```python
from build123d import *

# Parameters (mm, degrees)
ESQUISSE1_R                  = 7.5
BOSS_EXTRU_1_DEPTH           = 10
ESQUISSE1_5_R                = 14
ENL_V_MAT_EXTRU_1_DEPTH      = 2
ENL_V_MAT_EXTRU_1_DEPTH_BACK = 10
BOSS_EXTRU_2_DEPTH           = 45
ENL_V_MAT_EXTRU_2_DEPTH      = 11
ENL_V_MAT_EXTRU_2_DEPTH_BACK = 5


with BuildPart() as part:
    # Esquisse1 → Boss.-Extru.1 (new body, symmetric)
    with BuildSketch(Plane.XY):
        with BuildLine():
            Line((-634.508066615, 20.5), (-595.008671928, 20.5))
            Line((-595.008671928, 20.5), (-595.008671928, -24.5))
            Line((-595.008671928, -24.5), (-634.508066615, -24.5))
            ThreePointArc((-634.508066615, -24.5), (-657.008066615, -2), (-634.508066615, 20.5))
        make_face()
        with Locations((-634.508066615, -2)):
            Circle(ESQUISSE1_R, mode=Mode.SUBTRACT)
    extrude(amount=BOSS_EXTRU_1_DEPTH, both=True)

    # Esquisse1_5 → Enl_v. mat.-Extru.1 (cut, two sides)
    with BuildSketch(Plane.XY) as enl_v_mat_extru_1_sk:
        with Locations((-634.508066615, -2)):
            Circle(ESQUISSE1_5_R)
    extrude(amount=ENL_V_MAT_EXTRU_1_DEPTH, mode=Mode.SUBTRACT)
    extrude(enl_v_mat_extru_1_sk.sketch, amount=-ENL_V_MAT_EXTRU_1_DEPTH_BACK, mode=Mode.SUBTRACT)

    # Esquisse2 → Boss.-Extru.2 (add)
    with BuildSketch(Plane(origin=(0, 20.5, 0), x_dir=(1, 0, 0), z_dir=(0, 1, 0))):
        Polygon((-605.008671928, 10), (-605.008671928, 15), (-600.008671928, 15), (-600.008671928, 20), (-620.008671928, 20), (-620.008671928, 15), (-615.008671928, 15), (-615.008671928, 10), align=None)
    extrude(amount=-BOSS_EXTRU_2_DEPTH)

    # Esquisse1_7 → Enl_v. mat.-Extru.2 (cut, two sides)
    with BuildSketch(Plane.XY) as enl_v_mat_extru_2_sk:
        Polygon((-607.008671928, 20.5), (-613.008671928, 20.5), (-613.008671928, 18.5), (-615.008671928, 18.5), (-615.008671928, 16.5), (-605.008671928, 16.5), (-605.008671928, 18.5), (-607.008671928, 18.5), align=None)
    extrude(amount=ENL_V_MAT_EXTRU_2_DEPTH, mode=Mode.SUBTRACT)
    extrude(enl_v_mat_extru_2_sk.sketch, amount=-ENL_V_MAT_EXTRU_2_DEPTH_BACK, mode=Mode.SUBTRACT)


solid = part.part
```
For this review, take the finished solid that the model builds, in its own axes (mm). A direction names the side the tool comes from. Coordinates: 2 decimals unless noted, no trailing zeros. Write each loop counter-clockwise with the first axis right and the second up, starting at its lowest first coordinate (ties: lowest second). Pieces come first, ordered by that corner, then holes. Notation, with made-up numbers: (-18, 75) - (-10, 75) arc R17 ccw to (-10, 108) - close; hole circle Ø5 at (57.5, 5.5). An arc over 180 degrees is marked (long way). Put each result on its own line as item: value.
1. Add section D-D, the plane z = 4. Give the boundary of the cut face in (x, y), then the cut area to 3 significant figures.
Values found:
outline: (-634.51, -24.5) - (-595.01, -24.5) - (-595.01, 20.5) - (-607.01, 20.5) - (-607.01, 18.5) - (-605.01, 18.5) - (-605.01, 16.5) - (-615.01, 16.5) - (-615.01, 18.5) - (-613.01, 18.5) - (-613.01, 20.5) - (-634.51, 20.5) arc R22.5 ccw to start; hole circle Ø15 at (-634.51, -2)
area: 2,360 mm²
2. Add section A-A, the plane z = 0.5. Give the boundary of the cut face in (x, y), then the cut area to 3 significant figures.
Values found:
outline: (-634.51, -24.5) - (-595.01, -24.5) - (-595.01, 20.5) - (-607.01, 20.5) - (-607.01, 18.5) - (-605.01, 18.5) - (-605.01, 16.5) - (-615.01, 16.5) - (-615.01, 18.5) - (-613.01, 18.5) - (-613.01, 20.5) - (-634.51, 20.5) arc R22.5 ccw to start; hole circle Ø28 at (-634.51, -2)
area: 1,920 mm²
3. Add section C-C, the plane x = -645. Give the boundary of the cut face in (y, z).
Values found:
outline: (-21.9, -10) - (-11.27, -10) - (-11.27, 2) - (7.27, 2) - (7.27, -10) - (17.9, -10) - (17.9, 10) - (-21.9, 10) - close
4. Wall thickness on probe 1 along Z at (x, y) = (-649.5, -13.5); probe 2 along Z at (x, y) = (-602, -20.5); probe 3 along X at (y, z) = (17.5, -10.5): over which ranges is each line inside the solid? List them lowest first.
Values found:
probe 1: -10 to 10
probe 2: -20 to -15, -10 to 10
probe 3: -615.01 to -605.01
5. Mouldability with a two-part tool opening along Y and no side actions: class faces 4 (the cylindrical face through (-657.003, -2.495, 0.14)), 5 (the flat face through (-610, 18, -5)), 6 (the flat face through (-615.009, 18, 2)), 7 (the flat face through (-645, -12, -10)) as released by +Y, released by -Y, zero draft, split by the parting line, or undercut.
Values found:
face 4: split by the parting line
face 5: undercut
face 6: undercut
face 7: zero draft
6. Machinability: for faces 1 (the cylindrical face through (-648.495, -1.384, -4.084)), 2 (the flat face through (-607.009, 19, 3)), 3 (the flat face through (-603, -2, -15)), which of the approach directions +Z, -Z, +X, -X, +Y, -Y give a long, thin tool a straight path to every point of the face, cutting with its end or side? Answer none if there is none.
Values found:
face 1: -Z
face 2: +Z, +Y
face 3: +X, +Y, -Y
7. Add section B-B, the plane y = -2. Give the boundary of the cut face in (x, z).
Values found:
outline: (-657.01, -10) - (-648.51, -10) - (-648.51, 2) - (-642.01, 2) - (-642.01, 10) - (-657.01, 10) - close; (-627.01, 2) - (-620.51, 2) - (-620.51, -10) - (-615.01, -10) - (-615.01, -15) - (-620.01, -15) - (-620.01, -20) - (-600.01, -20) - (-600.01, -15) - (-605.01, -15) - (-605.01, -10) - (-595.01, -10) - (-595.01, 10) - (-627.01, 10) - close
8. For pin 1 (2.5 mm diameter, centred on y = -2, z = -18.5, fed in from -X); pin 2 (5.5 mm diameter, centred on y = -8.5, z = -12.5, fed in from -X); pin 3 (1.5 mm diameter, centred on x = -626.5, y = 10.5, fed in from -Z), all flat-tipped, find the tip position at first contact; note any pin that passes through.
Values found:
pin 1: x = -620.01
pin 2: x = -656.36
pin 3: z = -10
